```python
from build123d import *

# Parameters (mm, degrees)
SKETCH1_R           = 25
BOSS_EXTRUDE1_DEPTH = 45
SKETCH2_R           = 2
CUT_EXTRUDE1_DEPTH  = 10
SKETCH3_R           = 3
BOSS_EXTRUDE2_DEPTH = 22
SKETCH4_R           = 1.5
CUT_EXTRUDE2_DEPTH  = 10
BOSS_EXTRUDE3_START = 2
SKETCH5_R           = 3
BOSS_EXTRUDE3_DEPTH = 2
CHAMFER1_SIZE       = 3


with BuildPart() as part:
    # Sketch1 → Boss-Extrude1 (new body)
    with BuildSketch(Plane.XY):
        with Locations(Location((0, 0, 0), (0, 0, 180))):
            Circle(SKETCH1_R)
    extrude(amount=BOSS_EXTRUDE1_DEPTH)

    # Sketch2 → Cut-Extrude1 (cut)
    with BuildSketch(Plane.XY.offset(45)):
        with Locations((0, 15)):
            Circle(SKETCH2_R)
        with Locations(Location((0, -15, 0), (0, 0, 180))):
            Circle(SKETCH2_R)
        with Locations((-15, 0)):
            Circle(SKETCH2_R)
        with Locations(Location((15, 0, 0), (0, 0, 180))):
            Circle(SKETCH2_R)
    extrude(amount=-CUT_EXTRUDE1_DEPTH, mode=Mode.SUBTRACT)

    # Sketch3 → Boss-Extrude2 (add)
    with BuildSketch(Plane.XY.offset(45)):
        Circle(SKETCH3_R)
    extrude(amount=BOSS_EXTRUDE2_DEPTH)

    # Sketch4 → Cut-Extrude2 (cut)
    with BuildSketch(Plane(origin=(0, 0, 0), x_dir=(-1, 0, 0), z_dir=(0, 0, -1))):
        with Locations((0, 10)):
            Circle(SKETCH4_R)
        with Locations(Location((0, -10, 0), (0, 0, 180))):
            Circle(SKETCH4_R)
        with Locations((-10, 0)):
            Circle(SKETCH4_R)
        with Locations(Location((10, 0, 0), (0, 0, 180))):
            Circle(SKETCH4_R)
    extrude(amount=-CUT_EXTRUDE2_DEPTH, mode=Mode.SUBTRACT)

    # Sketch5 → Boss-Extrude3 (add)
    with BuildSketch(Plane(origin=(0, 0, 0), x_dir=(-1, 0, 0), z_dir=(0, 0, -1)).offset(BOSS_EXTRUDE3_START)):
        with Locations(Location((0, 0, 0), (0, 0, 180))):
            Circle(SKETCH5_R)
    extrude(amount=-BOSS_EXTRUDE3_DEPTH)

    # Chamfer1
    chamfer1_edges = [part.edges().sort_by_distance(p)[0] for p in [
        (25, 0, 0),
    ]]
    chamfer(chamfer1_edges, length=CHAMFER1_SIZE)


solid = part.part
```
The model under review builds one solid part; all positions refer to its coordinate system, in mm. A direction names the side the tool comes from. Round coordinates to 2 decimals unless told otherwise and drop trailing zeros. Write each loop counter-clockwise with the first axis right and the second up, starting at its lowest first coordinate (ties: lowest second). Pieces come first, ordered by that corner, then holes.
(1) We need section D-D on z = 57.5. Give the boundary of the cut face in (x, y), and give its area (3 significant figures).
(2) We need section C-C on z = 32. Give the boundary of the cut face in (x, y).
(3) Machinability: for faces 4 (the flat face through (-10, 0, 10)), 5 (the flat face through (15, 0, 35)), 6 (the flat face through (0, 0, -2)), which of the approach directions +Z, -Z, +X, -X, +Y, -Y give a long, thin tool a straight path to every point of the face, cutting with its end or side? Answer none if there is none.
(4) Mouldability with a two-part tool opening along Y and no side actions: class faces 1 (the flat face through (0, 5, 45)), 2 (the flat face through (0, 10, 10)), 3 (the cylindrical face through (-23.846, -7.509, 23.706)) as +Y half, -Y half, draft (parallel to the pull), parting line (faces both ways), or undercut.
(5) We need section A-A on z = 4. Give the boundary of the cut face in (x, y), and give its area (3 significant figures).
(6) Insertion check: pin 1 (4 mm diameter, centred on x = 5.5, y = 16.5, fed in from +Z); pin 2 (8 mm diameter, centred on y = 15, z = 11.5, fed in from -X); pin 3 (3 mm diameter, centred on x = -15, y = 0, fed in from +Z). Each pin has a flat end and moves straight along its axis. Give the tip position at first contact, or say it passes through.
(7) Wall thickness on L1, parallel to Y at x = 0, z = 5.75; L2, parallel to Z at x = -16.5, y = -9; L3, parallel to X at y = 16, z = 42: over which ranges is each line inside the solid? List them lowest first.
Findings below:
1. outline: circle Ø6 at (0, 0)
1. area: 28.3 mm2
2. outline: circle Ø50 at (0, 0)
3. face 4: -Z
3. face 5: +Z
3. face 6: -Z, +X, -X, +Y, -Y
4. face 1: draft
4. face 2: undercut
4. face 3: parting line
5. outline: circle Ø50 at (0, 0); hole circle Ø3 at (-10, 0); hole circle Ø3 at (0, -10); hole circle Ø3 at (0, 10); hole circle Ø3 at (10, 0)
5. area: 1,940 mm2
6. pin 1: stops at z = 45
6. pin 2: stops at x = -22.45
6. pin 3: stops at z = 35
7. L1: y = -25 to -11.5, -8.5 to 8.5, 11.5 to 25
7. L2: z = 0 to 45
7. L3: x = -19.21 to -1.73, 1.73 to 19.21
